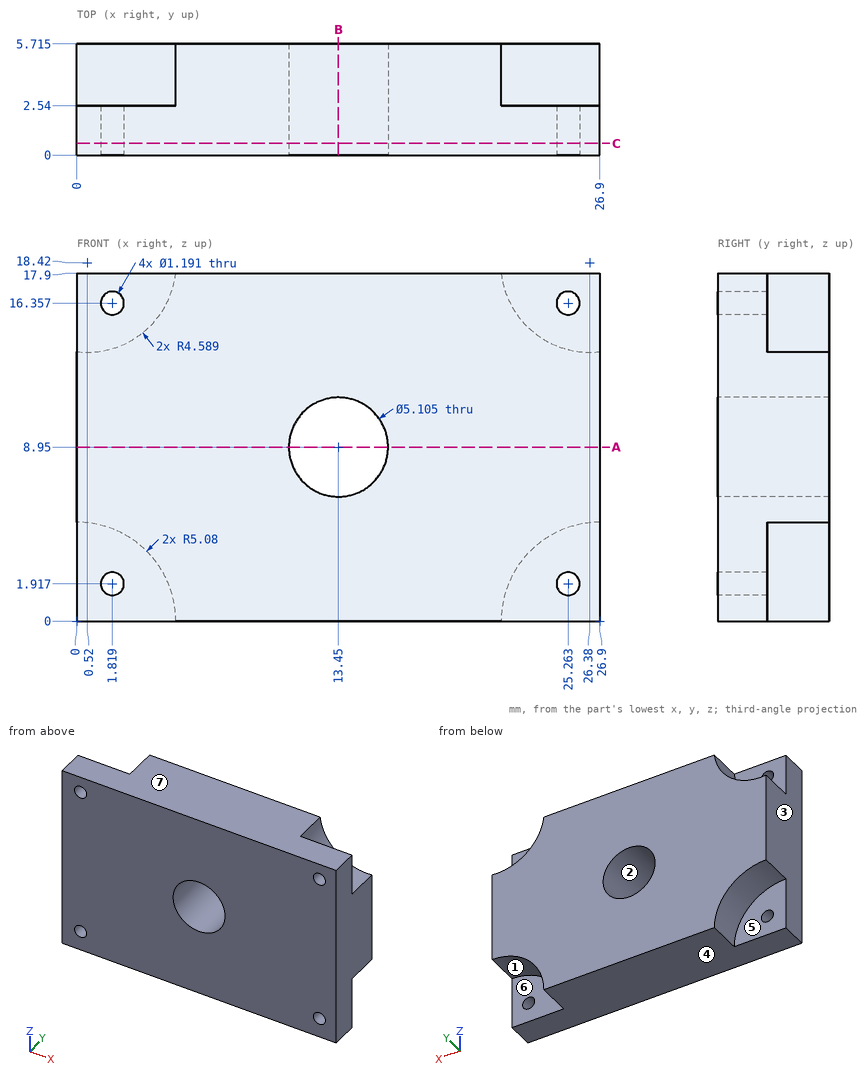
Check sheet for the drawn part. Datum: minimum x, y, z corner. Units: mm. A direction names the side the tool comes from. Coordinates: 2 decimals unless noted, no trailing zeros. Loops run counter-clockwise (first coordinate to the right, second up) from the corner with the lowest first, then second, coordinate; pieces in that order, holes last. Notation, with made-up numbers: (29, 74) -> (81, 74) arc R12 cw to (81, 88) -> close; hole circle Ø2 at (32.5, 0.25). An arc over 180 degrees is marked (long way). Answer in a Markdown table with one row per item.
1) Scan lines: line 1 along Z through (x, y) = (13.45, 1.9); line 2 along Y through (x, z) = (25.75, 4); line 3 along X through (y, z) = (3.45, 9). Record each from-to range of solid material in increasing order. Write a range as from..to.
The answers:
| item | result |
|---|---|
| line 1 | z = 0..6.4, 11.5..17.9 |
| line 2 | y = 0..2.54 |
| line 3 | x = 0..10.9, 16..26.9 |
2) Draft check along X on the marked faces 1, 2, 3 and 4. Enter one of: released by +X, released by -X, zero draft, split by the parting line, or undercut.
The answers:
| item | result |
|---|---|
| face 1 | released by +X |
| face 2 | undercut |
| face 3 | released by -X |
| face 4 | zero draft |
3) Section check A-A (z = 8.95). Record the cut outline in (x, y) (1 decimal).
The answers:
| item | result |
|---|---|
| outline | (0, 0) -> (10.9, 0) -> (10.9, 5.7) -> (0, 5.7) -> close; (16, 0) -> (26.9, 0) -> (26.9, 5.7) -> (16, 5.7) -> close |
4) Access from +Z, -Z, +X, -X, +Y, -Y to the whole of each face (thin tool, end or side, straight path). Record for the marked faces 5, 6 and 7.
The answers:
| item | result |
|---|---|
| face 5 | -Z, -X, +Y |
| face 6 | -Z, +X, +Y |
| face 7 | +Z, +X, -X, +Y, -Y |
5) Section check B-B (x = 13.45). Record the cut outline in (y, z) (1 decimal).
The answers:
| item | result |
|---|---|
| outline | (0, 0) -> (5.7, 0) -> (5.7, 6.4) -> (0, 6.4) -> close; (0, 11.5) -> (5.7, 11.5) -> (5.7, 17.9) -> (0, 17.9) -> close |
6) Depth check by flat-ended pin: P1, Ø1.5, axis at x = 1.82, z = 16.36, coming from the +Y side; P2, Ø2, axis at x = 3, y = 4.5, coming from the +Z side. Enter the tip coordinate at first touch or a pass-through.
The answers:
| item | result |
|---|---|
| P1 | stops at y = 2.54 |
| P2 | stops at z = 15.43 |
7) Section check C-C (y = 0.6). Give the number of separate pieces and of enclosed holes in the cut face.
The answers:
| item | result |
|---|---|
| separate pieces | 1 |
| enclosed holes | 5 |
